For this review, take the finished solid that the model builds, in its own axes (mm). A direction names the side the tool comes from. Coordinates: 2 decimals unless noted, no trailing zeros. Write each loop counter-clockwise with the first axis right and the second up, starting at its lowest first coordinate (ties: lowest second). Pieces come first, ordered by that corner, then holes. Notation, with made-up numbers: (-30.75, -29.75) - (22.25, -29.75) arc R25 cw to (22.25, 2.25) - close; hole circle Ø1 at (12, 79). An arc over 180 degrees is marked (long way). Use one line per item in the form item = value. Start each with the question number.
1) Mouldability with a two-part tool opening along Y and no side actions: class faces 1 (the cylindrical face through (-30.789, 34.196, 2.465)), 2 (the flat face through (25, 32.5, 3)), 3 (the flat face through (25.805, 27.249, 5.542)) as pulls with the +Y half, pulls with the -Y half, needs draft (parallel to the pull), parting line crosses it, or undercut.
2) Tool access review of faces 4 (the flat face through (25.805, -32.751, 5.542)), 5 (the flat face through (26, -32.5, 3)): name each direction out of +Z, -Z, +X, -X, +Y, -Y from which nothing blocks a thin tool from reaching the whole face with its end or side.
3) We need section A-A (y = 16). Give the boundary of the cut face in (x, z), plus the area to 3 significant figures.
4) We need section C-C (x = 7). Give the boundary of the cut face in (y, z) (3 decimals), plus the area to 3 significant figures.
5) Insertion check: P1, Ø19.5, axis at x = -8, y = 6, coming from the +Z side; P2, Ø4, axis at x = -25, y = -15.5, coming from the +Z side. Each pin has a flat end and moves straight along its axis. Give the tip position at first contact, or say it passes through.
6) We need section B-B (z = 3.5). Give the boundary of the cut face in (x, y), plus the area to 3 significant figures.
7) We need section D-D (y = 31). Give the boundary of the cut face in (x, z).
8) For L1, parallel to Y at x = -26.5, z = 2.25; L2, parallel to Y at x = -0.5, z = 2.5; L3, parallel to Z at x = 15, y = -22, list the stretches that pass through material, from the lowest coordinate up. Write a range as from..to.
```python
from build123d import *

# Parameters (mm, degrees)
F0_W        = 65
F0_H        = 72
F0_R        = 2.5
F0_R_2      = 20
F1_DEPTH    = 5
F3_DEPTH    = 1.1
F5_DEPTH    = 72.001
F6_T1_DEPTH = 35


# Not quite as in the source:
# - a fillet or chamfer that OpenCascade refuses, or shapes differently, is made with other operations: its cross-section is extruded or revolved along the edge and cut away or added


with BuildPart() as f1:
    # F0 (on Top) → F1 (new body)
    with BuildSketch(Plane.XY):
        Rectangle(F0_W, F0_H)
        with Locations((-26.5, -30)):
            Circle(F0_R, mode=Mode.SUBTRACT)
        with BuildLine():
            Line((26.5, -32.5), (24.5, -32.5))
            ThreePointArc((24.5, -32.5), (22, -30), (24.5, -27.5))
            Line((24.5, -27.5), (26.5, -27.5))
            ThreePointArc((26.5, -27.5), (29, -30), (26.5, -32.5))
        make_face(mode=Mode.SUBTRACT)
        with Locations((-26.5, 30)):
            Circle(F0_R, mode=Mode.SUBTRACT)
        Circle(F0_R_2, mode=Mode.SUBTRACT)
        with BuildLine():
            Line((26.5, 27.5), (24.5, 27.5))
            ThreePointArc((24.5, 27.5), (22, 30), (24.5, 32.5))
            Line((24.5, 32.5), (26.5, 32.5))
            ThreePointArc((26.5, 32.5), (29, 30), (26.5, 27.5))
        make_face(mode=Mode.SUBTRACT)
    extrude(amount=F1_DEPTH)

    # F2 (on face) → F3 (join)
    with BuildSketch(Plane.XY.offset(5)):
        with BuildLine():
            Line((26.5, -24.0000002086), (24.5, -24.0000002086))
            ThreePointArc((24.5, -24.0000002086), (18.5000002086, -30), (24.5, -35.9999997914))
            Line((24.5, -35.9999997914), (26.5, -35.9999997914))
            ThreePointArc((26.5, -35.9999997914), (30.7426405396, -34.2426405396), (32.4999997914, -30))
            ThreePointArc((32.4999997914, -30), (30.7426405396, -25.7573594604), (26.5, -24.0000002086))
        make_face()
        with BuildLine():
            ThreePointArc((26.5, -27.5), (29, -30), (26.5, -32.5))
            Line((26.5, -32.5), (24.5, -32.5))
            ThreePointArc((24.5, -32.5), (22, -30), (24.5, -27.5))
            Line((24.5, -27.5), (26.5, -27.5))
        make_face(mode=Mode.SUBTRACT)
        with BuildLine():
            ThreePointArc((26.5, 24.0000002086), (30.7426405396, 25.7573594604), (32.4999997914, 30))
            ThreePointArc((32.4999997914, 30), (30.7426405396, 34.2426405396), (26.5, 35.9999997914))
            Line((26.5, 35.9999997914), (24.5, 35.9999997914))
            ThreePointArc((24.5, 35.9999997914), (18.5000002086, 30), (24.5, 24.0000002086))
            Line((24.5, 24.0000002086), (26.5, 24.0000002086))
        make_face()
        with BuildLine():
            ThreePointArc((26.5, 32.5), (29, 30), (26.5, 27.5))
            Line((26.5, 27.5), (24.5, 27.5))
            ThreePointArc((24.5, 27.5), (22, 30), (24.5, 32.5))
            Line((24.5, 32.5), (26.5, 32.5))
        make_face(mode=Mode.SUBTRACT)
    extrude(amount=F3_DEPTH)

    # F4 (on face) → F5 (cut, through all)
    with BuildSketch(Plane.XZ.offset(36)):
        Polygon((19.295739324, 5), (32.5, 6.1), (18.5000002086, 6.1), (18.5000002086, 5), align=None)
    extrude(amount=-F5_DEPTH, mode=Mode.SUBTRACT)

    # F6: fillet of radius 6 on 4 edges, made by hand

    # F6_s2 → F6_t1 (cut)
    with BuildSketch(Plane.XY.offset(-15)):
        with BuildLine():
            ThreePointArc((-32.5, -30), (-30.7426406871, -34.2426406871), (-26.5, -36))
            Line((-26.5, -36), (-32.5, -36))
            Line((-32.5, -36), (-32.5, -30))
        make_face()
        with BuildLine():
            ThreePointArc((-32.5, 30), (-30.7426406871, 34.2426406871), (-26.5, 36))
            Line((-26.5, 36), (-32.5, 36))
            Line((-32.5, 36), (-32.5, 30))
        make_face()
        with BuildLine():
            ThreePointArc((32.5, 30), (30.7426406871, 34.2426406871), (26.5, 36))
            Line((26.5, 36), (32.5, 36))
            Line((32.5, 36), (32.5, 30))
        make_face()
        with BuildLine():
            ThreePointArc((32.5, -30), (30.7426406871, -34.2426406871), (26.5, -36))
            Line((26.5, -36), (32.5, -36))
            Line((32.5, -36), (32.5, -30))
        make_face()
    extrude(amount=F6_T1_DEPTH, mode=Mode.SUBTRACT)


solid = f1.part
```
Determined:
q1.face_1 = pulls with the +Y half
q1.face_2 = undercut
q1.face_3 = needs draft
q2.face_4 = +Z, -X, +Y, -Y
q2.face_5 = +Z, -Z
q3.outline = (-32.5, 0) - (-12, 0) - (-12, 5) - (-32.5, 5) - close; (12, 0) - (32.5, 0) - (32.5, 5) - (12, 5) - close
q3.area = 205 mm²
q4.outline = (-36, 0) - (-18.735, 0) - (-18.735, 5) - (-36, 5) - close; (18.735, 0) - (36, 0) - (36, 5) - (18.735, 5) - close
q4.area = 173 mm²
q5.P1 = through
q5.P2 = 5
q6.outline = (-32.5, -30) arc R6 ccw to (-26.5, -36) - (26.5, -36) arc R6 ccw to (32.5, -30) - (32.5, 30) arc R6 ccw to (26.5, 36) - (-26.5, 36) arc R6 ccw to (-32.5, 30) - close; hole circle Ø5 at (-26.5, -30); hole circle Ø5 at (-26.5, 30); hole circle Ø40 at (0, 0); hole (24.5, -32.5) - (26.5, -32.5) arc R2.5 ccw to (26.5, -27.5) - (24.5, -27.5) arc R2.5 ccw to start; hole (24.5, 27.5) - (26.5, 27.5) arc R2.5 ccw to (26.5, 32.5) - (24.5, 32.5) arc R2.5 ccw to start
q6.area = 3,290 mm²
q7.outline = (-32.42, 0) - (-28.79, 0) - (-28.79, 5) - (-32.42, 5) - close; (-24.21, 0) - (22.21, 0) - (22.21, 5.24) - (19.3, 5) - (-24.21, 5) - close; (28.79, 0) - (32.42, 0) - (32.42, 6.09) - (28.79, 5.79) - close
q8.L1 = -36..-32.5, -27.5..27.5, 32.5..36
q8.L2 = -36..-19.99, 19.99..36
q8.L3 = 0..5
